Could you check a few things on this model? Use its own coordinates, in mm. Face numbers are marked on the shaded views. A direction names the side the tool comes from. Coordinates: 2 decimals unless noted, no trailing zeros. Loops run counter-clockwise (first coordinate to the right, second up) from the corner with the lowest first, then second, coordinate; pieces in that order, holes last. Notation, with made-up numbers: M 89.5,-31.5 L 107.5,-31.5 A24 cw 107.5,-21.5 Z; hole C 71,25 d9. An arc over 180 degrees is marked long. Write each question's results on one line, items separated by ' | '.
Autodesk Inventor part; units mm, degrees
ref_plane "YZ Plane" through (0, 0, 0) normal (1, 0, 0) x (0, 1, 0)
ref_plane "XZ Plane" through (0, 0, 0) normal (0, 1, 0) x (-1, 0, 0)
ref_plane "XY Plane" through (0, 0, 0) normal (0, 0, 1) x (1, 0, 0)
sketch "Sketch1" plane through (0, 0, 0) normal (0, 0, 1) x (1, 0, 0)
  line L0 (0, 0) -> (25, 0)
  line L1 (25, 0) -> (25, 40)
  line L2 (25, 40) -> (0, 40)
  line L3 (0, 40) -> (0, 0)
  dimension "d1" = 25
  dimension "d2" = 40
  dimension "d3" = 25
extrude "Extrusion1" add sketch "Sketch1" against normal blind 30
sketch "Sketch2" plane through (25, 0, 0) normal (1, 0, 0) x (0, 0, -1)
  line L0 (0, 0) -> (30, 0)
  circle A0 centre (15, 6.56) radius 2.46
extrude "Extrusion2" cut sketch "Sketch2" against normal blind 30
sketch "Sketch3" plane through (0, 0, 0) normal (-1, 0, 0) x (0, 0, 1)
  line L0 (0, 0) -> (-30, 0)
  line L1 (-25.05, 0) -> (-4.95, 0)
  line L2 (-4.95, 0) -> (-4.95, 33.12)
  line L3 (-4.95, 33.12) -> (-25.05, 33.12)
  line L4 (-25.05, 33.12) -> (-25.05, 0)
  dimension "d11" = 20.1
extrude "Extrusion3" cut sketch "Sketch3" against normal blind 20
sketch "Sketch4" plane through (0, 0, 0) normal (0, -1, 0) x (1, 0, 0)
  line L0 (20, -4.95) -> (20, -25.05)
  line L1 (20, -15) -> (25, -15)
  line L2 (25, 0) -> (25, -30)
  line L3 (20, -8.025) -> (25, -8.025)
  line L4 (25, -8.025) -> (25, -21.975)
  line L5 (25, -21.975) -> (20, -21.975)
  line L6 (20, -21.975) -> (20, -8.025)
  line L7 (20, -8.025) -> (25, -21.975) construction
  line L8 (25, -8.025) -> (20, -21.975) construction
  line L9 (25, -12.54) -> (25, -17.46)
  point P0 (0, 0)
  point P1 (22.5, -15)
  dimension "d14" = 13.95
extrude "Extrusion4" add sketch "Sketch4" along normal blind 15
sketch "Sketch5" plane through (20, 0, 0) normal (-1, 0, 0) x (0, 0, 1)
  circle A0 centre (-15, 6.56) radius 2.46
  circle A1 centre (-15, 6.56) radius 4.7025
  circle A2 centre (-15, 6.56) radius 2.46
  circle A3 centre (-15, 6.56) radius 2.46
  point P0 (0, 0)
  dimension "d17" = 9.405
extrude "Extrusion5" cut sketch "Sketch5" against normal blind 2.1
sketch "Sketch6" plane through (25, 0, 0) normal (1, 0, 0) x (0, 0, -1)
  circle A0 centre (15, 6.56) radius 4.7025
  line L0 (15, 6.56) -> (15, 23.56)
  circle A1 centre (15, 23.56) radius 2.46
  point P0 (0, 0)
  dimension "d20" = 17
  dimension "d21" = 4.92
extrude "Extrusion6" cut sketch "Sketch6" against normal blind 10 contours A1
sketch "Sketch7" plane through (20, 0, 0) normal (-1, 0, 0) x (0, 0, 1)
  circle A0 centre (-15, 23.56) radius 2.46
  circle A1 centre (-15, 23.56) radius 4.7025
  point P0 (0, 0)
  dimension "d24" = 9.405
extrude "Extrusion7" cut sketch "Sketch7" against normal blind 2.1
sketch "Sketch9" plane through (25, 0, 0) normal (1, 0, 0) x (0, 0, -1)
  circle A0 centre (15, 6.56) radius 2.46
  circle A1 centre (15, 6.56) radius 2.46
  circle A2 centre (15, 23.56) radius 2.46
  circle A3 centre (15, 23.56) radius 2.46
  line L0 (30, 40) -> (30, 0)
  line L1 (30, 0) -> (30, 40)
  line L2 (30, 40) -> (0, 40)
  line L3 (0, 40) -> (0, 0)
  line L4 (0, 0) -> (8.025, 0)
  line L5 (21.975, 0) -> (21.975, -15)
  line L6 (21.975, -15) -> (8.025, -15)
  line L7 (8.025, -15) -> (8.025, 0)
  line L8 (0, 0) -> (8.025, 0)
  line L9 (21.975, 0) -> (30, 0)
extrude "Extrusion8" add sketch "Sketch9" along normal blind 5
sketch "Sketch10" plane through (0, 40, 0) normal (0, 1, 0) x (1, 0, 0)
  line L0 (0, 30) -> (30, 30)
  line L1 (30, 0) -> (0, 0)
  line L2 (0, 30) -> (30, 30)
  line L3 (30, 30) -> (30, 0)
  line L4 (30, 0) -> (0, 0)
  line L5 (0, 0) -> (0, 30)
extrude "Extrusion9" add sketch "Sketch10" along normal blind 30
sketch "Sketch12" plane through (30, 0, 0) normal (1, 0, 0) x (0, 0, -1)
  circle A0 centre (15, 6.56) radius 2.46
  line L0 (15, 6.56) -> (15, 15.06)
  circle A1 centre (15, 15.06) radius 2.525
  point P0 (0, 0)
  dimension "d31" = 8.5
  dimension "d33" = 5.05
extrude "Extrusion10" cut sketch "Sketch12" against normal blind 30 contours A1
sketch "Sketch15" plane through (0, 0, -25.05) normal (-1, 0, 0) x (0, 0, 1)
  line L0 (0, 33.12) -> (20.1, 33.12)
  line L1 (20.1, 33.12) -> (20.1, 0)
  line L2 (0, 33.12) -> (20.1, 33.12)
  line L3 (20.1, 33.12) -> (20.1, 31.1)
  line L4 (20.1, 31.1) -> (0, 31.1)
  line L5 (0, 31.1) -> (0, 33.12)
  point P0 (25.05, 0)
  dimension "d57" = 2.02
extrude "Extrusion13" add sketch "Sketch15" against normal blind 20
sketch "Sketch17" plane through (0, 0, 0) normal (0, 0, 1) x (1, 0, 0)
  line L0 (0, 70) -> (30, 70)
  line L1 (30, 70) -> (50.0622, 90.0622)
  line L2 (30, 70) -> (80, 70) construction
  line L3 (11.9522, 97.2454) -> (0, 85.2932)
  line L4 (0, 70) -> (0, 85.2932)
  line L5 (0, 70) -> (0, 0)
  line L6 (0, 70) -> (30, 70)
  line L7 (10.923, 112.2849) -> (0, 120.567)
  line L8 (50.0622, 105.3553) -> (50.0622, 120.567)
  line L9 (50.0622, 105.3553) -> (50.0622, 90.0622)
  arc A0 (11.9522, 97.2454) -> (10.923, 112.2849) centre (4.8811, 104.3165) ccw
  line L10 (0, 165.567) -> (30, 165.567)
  line L11 (30, 165.567) -> (50.0622, 120.567)
  line L12 (6, 163.067) -> (0, 165.567)
  line L13 (6, 123.067) -> (0, 120.567)
  line L14 (6, 123.067) -> (12, 143.067)
  line L15 (12, 143.067) -> (6, 163.067)
  dimension "d61" = 45
  dimension "d62" = 32.0271
  dimension "d72" = 10
extrude "Extrusion14" add sketch "Sketch17" against normal blind 30
properties part number "rec_c_40mm_x_30mm"
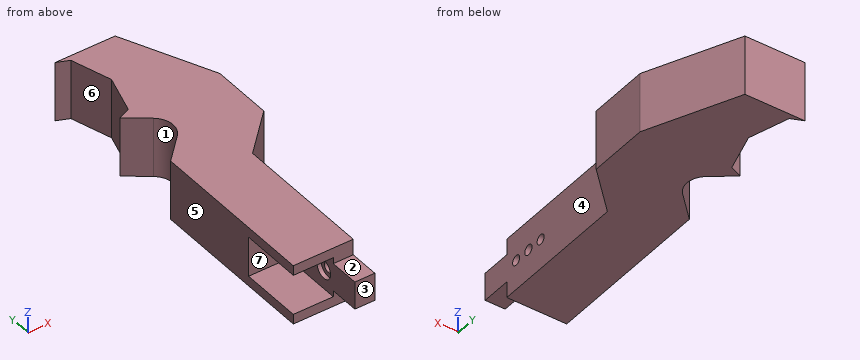
(1) Imagine slicing it at D-D, the plane y = 94. List the corners of the cut face in (x, z) for me.
Reported:
outline: M 8.71,-30 L 50.06,-30 L 50.06,0 L 8.71,0 Z
(2) If we mould it in two halves opening along Y, with no side actions, what happens to the marked faces 1, 2 and 3? For each: released by +Y, released by -Y, zero draft, split by the parting line, or undercut.
Reported:
face 1: undercut | face 2: zero draft | face 3: released by -Y
(3) Imagine slicing it at A-A, the plane y = 15.06. List the corners of the cut face in (x, z) for me (3 decimals).
Reported:
outline: M 0,-30 L 30,-30 L 30,-17.525 L 20,-17.525 L 20,-25.05 L 0,-25.05 Z; M 0,-4.95 L 20,-4.95 L 20,-12.475 L 30,-12.475 L 30,0 L 0,0 Z
(4) Imagine slicing it at C-C, the plane z = -15. State how many separate pieces and enclosed holes the cut face has, and give its area (3 significant figures).
Reported:
separate pieces: 4 | enclosed holes: 0 | area: 4,890 mm2
(5) Please list where these lines run through material, in increasing order: probe 1 along Y at (x, z) = (21.4, -15) (1 decimal); probe 2 along Y at (x, z) = (26, -15) (3 decimals); probe 3 along Z at (x, y) = (27, 6.56). Write a range as from..to.
Reported:
probe 1: y = -15..1.9, 11.3..12.5, 17.6..18.9, 28.3..165.6 | probe 2: y = -15..4.1, 9.02..12.535, 17.585..21.1, 26.02..165.567 | probe 3: z = -30..-17.46, -12.54..0
(6) Will these pins go through, and if not, where does the flat tip stop? P1, Ø9, axis at y = 35.5, z = -19, coming from the +X side; P2, Ø8, axis at y = 6.56, z = -15, coming from the -X side; P3, Ø9, axis at x = 12.5, z = -6, coming from the -Y side.
Reported:
P1: stops at x = 30 | P2: stops at x = 22.1 | P3: stops at y = 0
(7) Which directions (+Z, -Z, +X, -X, +Y, -Y) give clear straight access to the entire face, cutting with the end or side of a thin tool? Please do the marked faces 4, 5, 6 and 7.
Reported:
face 4: +Z, -Z, +X, -Y | face 5: +Z, -Z, -X, +Y, -Y | face 6: +Z, -Z, -X | face 7: -X, -Y
(8) Imagine slicing it at B-B, the plane x = 17. List the corners of the cut face in (y, z) for me, and give its area (3 significant figures).
Reported:
outline: M 0,-30 L 165.57,-30 L 165.57,0 L 0,0 L 0,-4.95 L 31.1,-4.95 L 31.1,-25.05 L 0,-25.05 Z | area: 4,340 mm2
